Read the model definition and answer for the solid it produces. Units are mm, in the model's axes. Face numbers are marked on the shaded views. A direction names the side the tool comes from. Round coordinates to 2 decimals unless told otherwise and drop trailing zeros. Write each loop counter-clockwise with the first axis right and the second up, starting at its lowest first coordinate (ties: lowest second). Pieces come first, ordered by that corner, then holes. Notation, with made-up numbers: (79.25, 33) -> (108.25, 33) arc R27 ccw to (108.25, 60) -> close; hole circle Ø1 at (26.5, 49). An arc over 180 degrees is marked (long way). Return JSON: item names as keys, results as strings.
from build123d import *

# Parameters (mm, degrees)
FILLET1_R             = 3
BOSS_EXTRUDE1_REACH   = 17.78
SKETCH3_W             = 6.625814586
SKETCH3_H             = 4
SKETCH2_W             = 30
SKETCH2_H             = 15
CUT_EXTRUDE1_DEPTH    = 18.320508133
F_3_0MM_DOWEL_HOLE1_D = 3
FILLET2_R             = 2


with BuildPart() as part:
    # Sketch1 → Revolve1 (revolve)
    with BuildSketch(Plane.XY):
        Polygon((2.25, 0), (2.25, 10), (3.75, 10), (3.75, 3), (10, 3), (10, 0), align=None)
    revolve(axis=Axis((0, -739.105470896, 0), (0, 1, 0)))

    # Fillet1
    fillet1_edges = [part.edges().sort_by_distance(p)[0] for p in [
        (-3.75, 3, 0),
    ]]
    fillet(fillet1_edges, radius=FILLET1_R)

    # Boss-Extrude1: up to this face of the body (flat: up to its plane)
    boss_extrude1_end = Plane(part.part.faces().sort_by_distance((-2.356066017, 10, 0))[0])
    # Sketch3 → Boss-Extrude1 (add, up to the picked face)
    with BuildSketch(Plane(origin=(0, 3, 0), x_dir=(1, 0, 0), z_dir=(0, 1, 0)), mode=Mode.PRIVATE) as boss_extrude1_sk1:
        with Locations((-6.485051678, 0)):
            Rectangle(SKETCH3_W, SKETCH3_H)
    boss_extrude1_tool1 = split(extrude(boss_extrude1_sk1.sketch, amount=BOSS_EXTRUDE1_REACH, mode=Mode.PRIVATE), bisect_by=boss_extrude1_end, keep=Keep.BOTH, mode=Mode.PRIVATE)
    boss_extrude1 = boss_extrude1_tool1.solids().sort_by(Axis((-6.485052, 3, 0), (0, 1, 0)))[0]
    add(boss_extrude1)

    # Mirror1: Boss-Extrude1 across plane
    add(boss_extrude1.mirror(Plane(origin=(0, 0, 0), x_dir=(0, 0, 1), z_dir=(1, 0, 0))))

    # Sketch2 → Cut-Extrude1 (cut, through all)
    with BuildSketch(Plane(origin=(0, 0, 0), x_dir=(1, 0, 0), z_dir=(0, 1, 0))):
        with Locations((0, -7.5)):
            Rectangle(SKETCH2_W, SKETCH2_H)
    extrude(amount=CUT_EXTRUDE1_DEPTH, mode=Mode.SUBTRACT)

    # Ø3.0mm Dowel Hole1 (through all)
    with Locations(Plane(origin=(0, 0, -2), x_dir=(-1, 0, 0), z_dir=(0, 0, -1))):
        with Locations((6.797958971, 7), (-6.797958971, 7)):
            Hole(F_3_0MM_DOWEL_HOLE1_D / 2)

    # Fillet2
    fillet2_edges = [part.edges().sort_by_distance(p)[0] for p in [
        (-9.797958971, 10, -1),
        (9.797958971, 10, -1),
    ]]
    fillet(fillet2_edges, radius=FILLET2_R)


solid = part.part
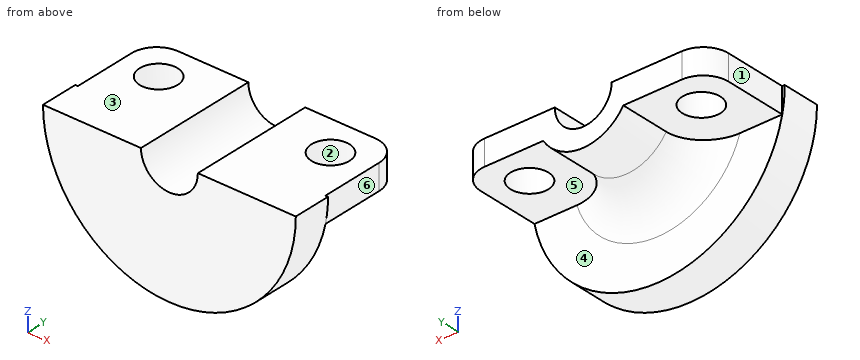
Item 1: Section C-C (x = 0) is taken. Give the vertices of the cut face in (y, z), then the cut area to 3 significant figures.
Worked answers:
{"outline": "(0, -10) -> (3, -10) -> (3, -6.75) arc R3 cw to (6, -3.75) -> (10, -3.75) -> (10, -2.25) -> (0, -2.25) -> close", "area": "35.7 mm2"}
Item 2: A tool of negligible diameter and unlimited length cuts with its end or side. For the marked faces 4, 5 and 6, from which of +Z, -Z, +X, -X, +Y, -Y can it reach the whole face along a straight path? Write none if from no direction.
Worked answers:
{"face 4": "-Z, +Y", "face 5": "-Z, +X, +Y", "face 6": "+Z, -Z, +X, +Y"}
Item 3: For a pull along X with two mould halves and no side action, classify the marked faces 1, 2 and 3 as released by +X, released by -X, zero draft, split by the parting line, or undercut.
Worked answers:
{"face 1": "released by -X", "face 2": "undercut", "face 3": "zero draft"}
Item 4: Straight lines are drawn through the part: L1, parallel to Y at x = -4.25, z = -6.75; L2, parallel to Z at x = 4, y = 9.25; L3, parallel to X at y = 9.25, z = -1.5. For each, find the intervals that lie inside material, in ascending order. Write a range as [from, to].
Worked answers:
{"L1": "y = [0, 3]", "L2": "z = [-2, 0]", "L3": "x = [-9.36, -1.68], [1.68, 9.36]"}
Item 5: Section B-B (z = -1.25) is taken. Give the vertices of the cut face in (x, y).
Worked answers:
{"outline": "(-9.92, 0) -> (-1.87, 0) -> (-1.87, 10) -> (-7.8, 10) arc R2 ccw to (-9.8, 8) -> (-9.8, 3) -> (-9.92, 3) -> close; (1.87, 0) -> (9.92, 0) -> (9.92, 3) -> (9.8, 3) -> (9.8, 8) arc R2 ccw to (7.8, 10) -> (1.87, 10) -> close; hole circle Ø3 at (-6.8, 7); hole circle Ø3 at (6.8, 7)"}
Item 6: Section D-D (y = 9) is taken. Give the vertices of the cut face in (x, z), then the cut area to 3 significant figures.
Worked answers:
{"outline": "(-9.53, -2) -> (-3.17, -2) arc R3.75 ccw to (3.17, -2) -> (9.53, -2) -> (9.53, 0) -> (2.25, 0) arc R2.25 cw to (-2.25, 0) -> (-9.53, 0) -> close", "area": "38.0 mm2"}
Item 7: Section A-A (y = 7) is taken. Give the vertices of the cut face in (x, z).
Worked answers:
{"outline": "(-9.8, -2) -> (-8.3, -2) -> (-8.3, 0) -> (-9.8, 0) -> close; (-5.3, -2) -> (-3.17, -2) arc R3.75 ccw to (3.17, -2) -> (5.3, -2) -> (5.3, 0) -> (2.25, 0) arc R2.25 cw to (-2.25, 0) -> (-5.3, 0) -> close; (8.3, -2) -> (9.8, -2) -> (9.8, 0) -> (8.3, 0) -> close"}
Item 8: Flat-ended cylindrical pins translate along their axes: pin 1 (1 mm diameter, centred on x = 6, z = -5, fed in from +Y); pin 2 (2 mm diameter, centred on y = 5.5, z = -1, fed in from -X); pin 3 (2.5 mm diameter, centred on x = 6.8, y = 7, fed in from -Z); pin 4 (1.5 mm diameter, centred on x = 3.5, y = 5, fed in from +Z). Find the tip coordinate at first contact, or state that the pin passes through.
Worked answers:
{"pin 1": "stops at y = 3", "pin 2": "stops at x = -9.8", "pin 3": "passes through", "pin 4": "stops at z = 0"}
